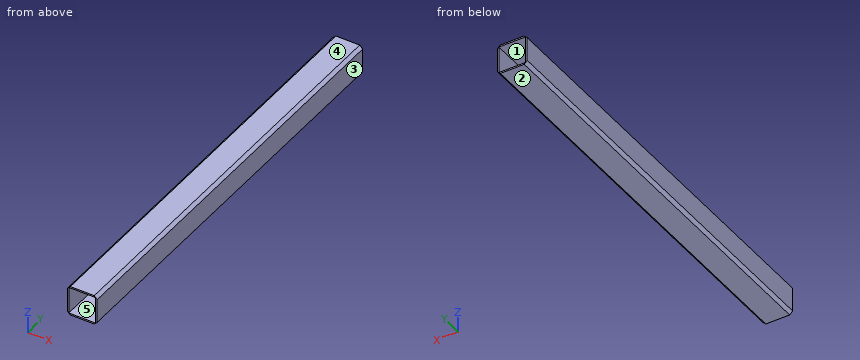
from build123d import *

# Parameters (mm, degrees)
SKETCH1_W           = 50
SKETCH1_H           = 700
BOSS_EXTRUDE1_DEPTH = 50
SKETCH2_W           = 45
SKETCH2_H           = 45
CUT_EXTRUDE1_DEPTH  = 704.562363974
CHAMFER5_SIZE       = 5


with BuildPart() as part:
    # Sketch1 → Boss-Extrude1 (new body)
    with BuildSketch(Plane.XY):
        with Locations((25, 350)):
            Rectangle(SKETCH1_W, SKETCH1_H)
    extrude(amount=BOSS_EXTRUDE1_DEPTH)

    # Sketch2 → Cut-Extrude1 (cut, through all)
    with BuildSketch(Plane(origin=(0, 700, 0), x_dir=(1, 0, 0), z_dir=(0, 1, 0))):
        with Locations((25, -25)):
            Rectangle(SKETCH2_W, SKETCH2_H)
    extrude(amount=-CUT_EXTRUDE1_DEPTH, mode=Mode.SUBTRACT)

    # Chamfer5
    chamfer5_edges = [part.edges().sort_by_distance(p)[0] for p in [
        (50, 350, 50),
        (0, 350, 50),
        (50, 350, 0),
        (0, 350, 0),
    ]]
    chamfer(chamfer5_edges, length=CHAMFER5_SIZE - 0.0001)  # a hair under: the kernel refuses the full size


solid = part.part
Verification items for the finished model (mm, model axes). Face numbers are marked on the shaded views. A direction names the side the tool comes from. Coordinates: 2 decimals unless noted, no trailing zeros. Order: outer loops, then holes, each group sorted by start corner. A loop starts at its lowest first (then second) coordinate and runs counter-clockwise, first axis right, second up. Notation, with made-up numbers: (19.5, -13.75) -> (61.5, -13.75) arc R6 ccw to (61.5, -2.75) -> close; hole circle Ø6 at (36, 43.5). An arc over 180 degrees is marked (long way). Put each result on its own line as item: value. Start each with the question number.
1. Cross-section at A-A, the plane y = 159. Record the boundary of the cut face in (x, z).
2. Material ranges on L1, parallel to X at y = 158, z = 33.5; L2, parallel to X at y = 455.5, z = 4, recorded low to high. Write a range as [from, to].
3. Mould release check, pull along Z, two halves, no side actions. Record for the marked faces 3, 4 and 5: released by +Z, released by -Z, zero draft, split by the parting line, or undercut.
4. Access from +Z, -Z, +X, -X, +Y, -Y to the whole of each face (thin tool, end or side, straight path). Record for the marked faces 1 and 2.
5. Cross-section at C-C, the plane z = 22. Record the boundary of the cut face in (x, y).
6. Cross-section at B-B, the plane x = 25.5. Record the boundary of the cut face in (y, z), then the cut area to 3 significant figures.
Computed:
1. outline: (0, 5) -> (5, 0) -> (45, 0) -> (50, 5) -> (50, 45) -> (45, 50) -> (5, 50) -> (0, 45) -> close; hole (2.5, 2.5) -> (47.5, 2.5) -> (47.5, 47.5) -> (2.5, 47.5) -> close
2. L1: [0, 2.5], [47.5, 50]
2. L2: [1, 2.5], [47.5, 49]
3. face 3: zero draft
3. face 4: released by +Z
3. face 5: undercut
4. face 1: +Y, -Y
4. face 2: -Z, +X, -X, +Y, -Y
5. outline: (0, 0) -> (2.5, 0) -> (2.5, 700) -> (0, 700) -> close; (47.5, 0) -> (50, 0) -> (50, 700) -> (47.5, 700) -> close
6. outline: (0, 0) -> (700, 0) -> (700, 2.5) -> (0, 2.5) -> close; (0, 47.5) -> (700, 47.5) -> (700, 50) -> (0, 50) -> close
6. area: 3,500 mm2
